```python
from build123d import *

# Parameters (mm, degrees)
F0_W      = 55
F0_H      = 20
F1_DEPTH  = 5
F2_R      = 4.8
F3_DEPTH  = 2.8
F4_R      = 2.625
F5_DEPTH  = 25
F2_R_2    = 1.55
F6_DEPTH  = 25
F8_DEPTH  = 2.45
F9_W      = 10
F9_H      = 5
F9_W_2    = 5.794909
F10_DEPTH = 2.5


with BuildPart() as f1:
    # F0 (on Top) → F1 (new body)
    with BuildSketch(Plane.XY):
        Rectangle(F0_W, F0_H)
    extrude(amount=F1_DEPTH)

    # F2 (on face) → F3 (cut)
    with BuildSketch(Plane.XY.offset(5)):
        Circle(F2_R)
    extrude(amount=-F3_DEPTH, mode=Mode.SUBTRACT)

    # F4 (on face) → F5 (cut)
    with BuildSketch(Plane(origin=(0, 0, 0), x_dir=(1, 0, 0), z_dir=(0, 0, -1))):
        Circle(F4_R)
    extrude(amount=-F5_DEPTH, mode=Mode.SUBTRACT)

    # F2 (on face) → F6 (cut)
    with BuildSketch(Plane.XY.offset(5)):
        with Locations((-17.5, 0)):
            Circle(F2_R_2)
        with Locations((17.5, 0)):
            Circle(F2_R_2)
    extrude(amount=-F6_DEPTH, mode=Mode.SUBTRACT)

    # F7 (on face) → F8 (cut)
    with BuildSketch(Plane(origin=(0, 0, 0), x_dir=(1, 0, 0), z_dir=(0, 0, -1))):
        Polygon((-16, 2.598076), (-19, 2.598076), (-20.5, 0), (-19, -2.598076), (-16, -2.598076), (-14.5, 0), align=None)
        Polygon((19, 2.598076), (16, 2.598076), (14.5, 0), (16, -2.598076), (19, -2.598076), (20.5, 0), align=None)
    extrude(amount=-F8_DEPTH, mode=Mode.SUBTRACT)

    # F9 (on face) → F10 (join)
    with BuildSketch(Plane(origin=(0, 0, 0), x_dir=(1, 0, 0), z_dir=(0, 0, -1))):
        Polygon((-27.5, 2.473653), (-27.5, -2.5), (-21.705, -2.526347), (-21.705, 2.473653), align=None)
        with Locations((-8.014056, -0.021072)):
            Rectangle(F9_W, F9_H)
        with Locations((8.194137, -0.011235)):
            Rectangle(F9_W, F9_H)
        with Locations((24.602545, 0)):
            Rectangle(F9_W_2, F9_H)
    extrude(amount=F10_DEPTH)


solid = f1.part
```
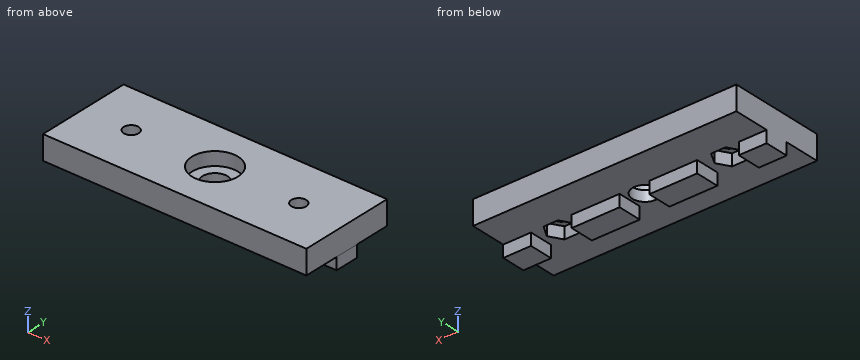
Part model, mm, in its own coordinate system. Round coordinates to 2 decimals unless told otherwise and drop trailing zeros. Order: outer loops, then holes, each group sorted by start corner. A loop starts at its lowest first (then second) coordinate and runs counter-clockwise, first axis right, second up. Notation, with made-up numbers: M 49.25,71 L 67.25,71 A25 cw 67.25,83 Z; hole C -12,-11.75 d3. An arc over 180 degrees is marked long. Put each result on its own line as item: value. Start each with the question number.
1. Slice it at C-C on z = 4.5. List the corners of the cut face in (x, y).
2. Slice it at B-B on x = 0. List the corners of the cut face in (y, z) (3 decimals).
3. Slice it at A-A on z = -1.5. List the corners of the cut face in (x, y) (3 decimals).
4. Drill centre lines: probe 1 along X at (y, z) = (0, 0.75) (3 decimals); probe 2 along Y at (x, z) = (17.5, 3.4); probe 3 along X at (y, z) = (-0.75, 2.25). Where is each one in solid material? Low to high. Write a range as [from, to].
5. Drop flat-ended pins along their axis: pin 1 (1.5 mm diameter, centred on x = 1.5, y = -1, fed in from -Z); pin 2 (4 mm diameter, centred on x = -17.5, y = 0.5, fed in from -Z); pin 3 (0.8 mm diameter, centred on x = 10.5, z = -1, fed in from +Y); pin 4 (1.2 mm diameter, centred on x = 24, z = -1.5, fed in from -Y). Give the stop position or say it passes through.
6. Slice it at D-D on x = -12. List the corners of the cut face in (y, z).
Findings:
1. outline: M -27.5,-10 L 27.5,-10 L 27.5,10 L -27.5,10 Z; hole C -17.5,0 d3.1; hole C 0,0 d9.6; hole C 17.5,0 d3.1
2. outline: M -10,0 L -2.625,0 L -2.625,2.2 L -4.8,2.2 L -4.8,5 L -10,5 Z; M 2.625,0 L 10,0 L 10,5 L 4.8,5 L 4.8,2.2 L 2.625,2.2 Z
3. outline: M -27.5,-2.474 L -21.705,-2.474 L -21.705,2.526 L -27.5,2.5 Z; M -13.014,-2.479 L -3.014,-2.479 L -3.014,2.521 L -13.014,2.521 Z; M 3.194,-2.489 L 13.194,-2.489 L 13.194,2.511 L 3.194,2.511 Z; M 21.705,-2.5 L 27.5,-2.5 L 27.5,2.5 L 21.705,2.5 Z
4. probe 1: [-27.5, -20.5], [-14.5, -2.625], [2.625, 14.5], [20.5, 27.5]
4. probe 2: [-10, -1.55], [1.55, 10]
4. probe 3: [-27.5, -20.07], [-14.93, -4.74], [4.74, 14.93], [20.07, 27.5]
5. pin 1: through
5. pin 2: z = 2.45
5. pin 3: y = 2.51
5. pin 4: y = -2.5
6. outline: M -10,0 L -2.48,0 L -2.48,-2.5 L 2.52,-2.5 L 2.52,0 L 10,0 L 10,5 L -10,5 Z
